Autodesk Inventor part; units mm, degrees
ref_plane "YZ Plane" through (0, 0, 0) normal (1, 0, 0) x (0, 1, 0)
ref_plane "XZ Plane" through (0, 0, 0) normal (0, 1, 0) x (-1, 0, 0)
ref_plane "XY Plane" through (0, 0, 0) normal (0, 0, 1) x (1, 0, 0)
sketch "Sketch1" plane through (0, 0, 0) normal (0, 0, 1) x (1, 0, 0)
  line L0 (0, 0) -> (1300, 0)
  line L1 (1300, 0) -> (1300, 50)
  line L2 (1300, 50) -> (0, 50)
  line L3 (0, 50) -> (0, 0)
  circle A0 centre (50, 25) radius 10.5
  circle A1 centre (1288, 40) radius 3
  circle A2 centre (1288, 10) radius 3
  line L4 (1182.5, 14.5) -> (1227.5, 14.5)
  line L5 (1227.5, 14.5) -> (1227.5, 35.5)
  line L6 (1227.5, 35.5) -> (1182.5, 35.5)
  line L7 (1182.5, 35.5) -> (1182.5, 14.5)
  circle A3 centre (14.5, 25) radius 5
  circle A4 centre (85.5, 25) radius 5
  dimension "d0" = 1300
  dimension "d1" = 50
  dimension "d2" = 21
  dimension "d3" = 6
  dimension "d4" = 6
  dimension "d5" = 45
  dimension "d6" = 21
  dimension "d7" = 14.5
  dimension "d8" = 72.5
  dimension "d13" = 10
  dimension "d14" = 10
extrude "Extrusion2" add sketch "Sketch1" along normal blind 6
equation "\"d7\" = -0.5 * d6 + 0.5 * d1"
properties part number "convyerwall2"
Read the model definition and answer for the solid it produces. Units are mm, in the model's axes. Round coordinates to 2 decimals unless told otherwise and drop trailing zeros. Write each loop counter-clockwise with the first axis right and the second up, starting at its lowest first coordinate (ties: lowest second). Pieces come first, ordered by that corner, then holes. Notation, with made-up numbers: (15.25, 34.5) -> (50.25, 34.5) arc R18 cw to (50.25, 41.5) -> close; hole circle Ø5 at (60, 14.25). An arc over 180 degrees is marked (long way). Answer in a Markdown table with one row per item. Add a question column.
1) Find section A-A, the plane z = 3.9. Determine the outline of the cut face in (x, y), and give its area (3 significant figures).
2) Determine the mould class of faces 1 (the face through (39.51, 24.54, 2.96)), 2 (the face through (641, 25, 0)) for opening direction Y: pulls with the +Y half, pulls with the -Y half, needs draft (parallel to the pull), parting line crosses it, or undercut.
3) Given P1, Ø9.5, axis at x = 1288, y = 40, coming from the +Z side, flat-ended and moving along its own axis, determine where the tip first touches the part or whether it passes through.
4) Consider line 1 (Y direction, x = 14.5, z = 4.1); line 2 (X direction, y = 9, z = 2.4); line 3 (X direction, y = 29, z = 0.8). Determine where each line is inside the solid, lowest interval first.
Findings below:
| question | item | result |
|---|---|---|
| 1 | outline | (0, 0) -> (1300, 0) -> (1300, 50) -> (0, 50) -> close; hole circle Ø10 at (14.5, 25); hole circle Ø21 at (50, 25); hole circle Ø10 at (85.5, 25); hole (1182.5, 14.5) -> (1227.5, 14.5) -> (1227.5, 35.5) -> (1182.5, 35.5) -> close; hole circle Ø6 at (1288, 10); hole circle Ø6 at (1288, 40) |
| 1 | area | 63,500 mm² |
| 2 | face 1 | undercut |
| 2 | face 2 | needs draft |
| 3 | P1 | z = 6 |
| 4 | line 1 | 0 to 20, 30 to 50 |
| 4 | line 2 | 0 to 1285.17, 1290.83 to 1300 |
| 4 | line 3 | 0 to 11.5, 17.5 to 40.29, 59.71 to 82.5, 88.5 to 1182.5, 1227.5 to 1300 |
